CAD build for the part. Positions are in the model's coordinates, mm. Face numbers are marked on the shaded views. A direction names the side the tool comes from. Coordinates: 2 decimals unless noted, no trailing zeros. Loops run counter-clockwise (first coordinate to the right, second up) from the corner with the lowest first, then second, coordinate; pieces in that order, holes last. Notation, with made-up numbers: (61, -10) -> (93, -10) arc R19 ccw to (93, -3) -> close; hole circle Ø6 at (18, 67.25). An arc over 180 degrees is marked (long way). Answer as CSV lines item,"result". Start each with the question number.
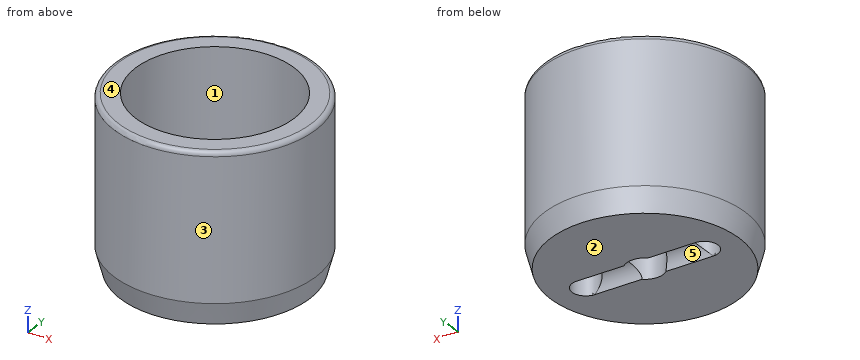
from build123d import *

# Parameters (mm, degrees)
F2_R     = 1.5
F3_DEPTH = 80
F4_R     = 0.5
F5_R     = 1.5
F6_DEPTH = 6.75


# Not quite as in the source:
# - a feature names something its author has since deleted; it is built from what else it names


with BuildPart() as f1:
    # F0 (on Front) → F1 (revolve)
    with BuildSketch(Plane.XZ):
        with BuildLine():
            Line((-8.65, 66), (-11, 66))
            Line((-11, 66), (-11, 50.0923395157))
            Line((-11, 50.0923395157), (-10.3264193874, 47.5785024464))
            Line((-10.3264193874, 47.5785024464), (-2, 47.5785024464))
            Line((-2, 47.5785024464), (-2, 50.8554930795))
            Line((-2, 50.8554930795), (-3, 53))
            Line((-3, 53), (-7.65, 53))
            ThreePointArc((-7.65, 53), (-8.3571067812, 53.2928932188), (-8.65, 54))
            Line((-8.65, 54), (-8.65, 66))
        make_face()
    revolve(axis=Axis((0, 0, 14.8610904367), (0, 0, -1)))

    # F2 (on Top) → F3 (cut)
    with BuildSketch(Plane.XY):
        with Locations((-6.5, 0)):
            Circle(F2_R)
        with BuildLine():
            ThreePointArc((8, 0), (6.5, 1.5), (5, 0))
            ThreePointArc((5, 0), (6.5, -1.5), (8, 0))
        make_face()
    extrude(amount=F3_DEPTH, mode=Mode.SUBTRACT)

    # F4
    f4_edges = [f1.edges().sort_by_distance(p)[0] for p in [
        (11, 0, 66),
    ]]
    fillet(f4_edges, radius=F4_R)

    # F5 (on Right) → F6 (cut, symmetric)
    with BuildSketch(Plane.YZ):
        with Locations((0, 47.5850664079)):
            Circle(F5_R)
    extrude(amount=F6_DEPTH, both=True, mode=Mode.SUBTRACT)


solid = f1.part
Item 1: Flat gauge pins, fed straight in: pin 1 Ø4 at (x, z) = (-5, 51.5) entering from +Y; pin 2 Ø6 at (y, z) = (-6.5, 57.5) entering from +X; pin 3 Ø2 at (y, z) = (-6.5, 52.5) entering from +X; pin 4 Ø10 at (y, z) = (1, 61.5) entering from +X. Where does each tip first touch, or does it go through?
Item 2: Saw through at B-B (x = 0). Write the cut outline in (y, z).
Item 3: Two-plate mould, pull along Y, no slides. Class the marked faces 3, 4 and 5: pulls with the +Y half, pulls with the -Y half, needs draft (parallel to the pull), parting line crosses it, or undercut.
Item 4: Wall check: probe 1 along Y at (x, z) = (0, 57); probe 2 along Z at (x, y) = (-2.25, 6.75). Give the ranges that are in metal, low to high.
Item 5: Which spindle directions (+Z, -Z, +X, -X, +Y, -Y) get a long thin tool onto all of the face, cutting with end or side? Do the marked faces 1 and 2. Say none if no direction does.
Item 6: Saw through at C-C (z = 61.25). Write the cut outline in (x, y), plus the area to 3 significant figures.
Item 7: Saw through at A-A (y = 0). Write the cut outline in (x, z).
Geometry check:
1,pin 1,"y = 10.58"
1,pin 2,"x = 10.43"
1,pin 3,"x = 9.53"
1,pin 4,"x = 11"
2,outline,"(-11, 50.09) -> (-10.33, 47.58) -> (-2, 47.58) -> (-2, 50.86) -> (-3, 53) -> (-7.65, 53) arc R1 cw to (-8.65, 54) -> (-8.65, 66) -> (-10.5, 66) arc R0.5 ccw to (-11, 65.5) -> close; (2, 47.58) -> (10.33, 47.58) -> (11, 50.09) -> (11, 65.5) arc R0.5 ccw to (10.5, 66) -> (8.65, 66) -> (8.65, 54) arc R1 cw to (7.65, 53) -> (3, 53) -> (2, 50.86) -> close"
3,face 3,"parting line crosses it"
3,face 4,"needs draft"
3,face 5,"undercut"
4,probe 1,"-11 to -8.65, 8.65 to 11"
4,probe 2,"47.58 to 53"
5,face 1,"+Z"
5,face 2,"-Z, +X, -X, +Y, -Y"
6,outline,"circle Ø22 at (0, 0); hole circle Ø17.3 at (0, 0)"
6,area,"145 mm2"
7,outline,"(-11, 50.09) -> (-10.33, 47.58) -> (-8, 47.58) -> (-8, 53.06) arc R1 cw to (-8.65, 54) -> (-8.65, 66) -> (-10.5, 66) arc R0.5 ccw to (-11, 65.5) -> close; (-5, 49.09) -> (-2, 49.09) -> (-2, 50.86) -> (-3, 53) -> (-5, 53) -> close; (2, 49.09) -> (5, 49.09) -> (5, 53) -> (3, 53) -> (2, 50.86) -> close; (8, 47.58) -> (10.33, 47.58) -> (11, 50.09) -> (11, 65.5) arc R0.5 ccw to (10.5, 66) -> (8.65, 66) -> (8.65, 54) arc R1 cw to (8, 53.06) -> close"
